from build123d import *

# Parameters (mm, degrees)
CYLINDER713_R     = 1.5
CYLINDER713_DEPTH = 14
CYLINDER710_R     = 1.5
CYLINDER710_DEPTH = 14
CYLINDER711_R     = 1.5
CYLINDER711_DEPTH = 14
CYLINDER712_R     = 1.5
CYLINDER712_DEPTH = 14
BOX045_W          = 15
BOX045_H          = 7.5
BOX045_DEPTH      = 2
BOX044_W          = 15
BOX044_H          = 20
BOX044_DEPTH      = 2
FILLET001008_R    = 3
BOX046_W          = 8
BOX046_H          = 9
BOX046_DEPTH      = 2


with BuildPart() as cylinder783:
    # Cylinder713 → Cylinder713 (new body)
    with BuildSketch(Plane(origin=(-4.5, -50.5, -7), x_dir=(1, 0, 0), z_dir=(0, 0, 1))):
        Circle(CYLINDER713_R)
    extrude(amount=CYLINDER713_DEPTH)


with BuildPart() as fusion001005002004004005002010_body:
    # Cylinder710 → Cylinder710 (new body)
    with BuildSketch(Plane(origin=(4.5, -50.5, -7), x_dir=(1, 0, 0), z_dir=(0, 0, 1))):
        Circle(CYLINDER710_R)
    extrude(amount=CYLINDER710_DEPTH)

    # Fusion001005002004004005002010002003003003017007024017: union Cylinder783
    add(cylinder783.part)


with BuildPart() as fusion001005002004004005002010_body_1:
    # Fusion001005002004004005002010002003003003017007024017 placement: moved
    add(fusion001005002004004005002010_body.part.moved(Location((0, 4, -3))))


with BuildPart() as cylinder781:
    # Cylinder711 → Cylinder711 (new body)
    with BuildSketch(Plane(origin=(-4.5, -50.5, -7), x_dir=(1, 0, 0), z_dir=(0, 0, 1))):
        Circle(CYLINDER711_R)
    extrude(amount=CYLINDER711_DEPTH)


with BuildPart() as fusion001005002004004005002010_body2:
    # Cylinder712 → Cylinder712 (new body)
    with BuildSketch(Plane(origin=(4.5, -50.5, -7), x_dir=(1, 0, 0), z_dir=(0, 0, 1))):
        Circle(CYLINDER712_R)
    extrude(amount=CYLINDER712_DEPTH)

    # Fusion001005002004004005002010002003003003017007024018: union Cylinder781
    add(cylinder781.part)


with BuildPart() as fusion001005002004004005002010_body2_1:
    # Fusion001005002004004005002010002003003003017007024018 placement: moved
    add(fusion001005002004004005002010_body2.part.moved(Location((0, 18, -3))))

    # Fusion001005002004004005002010002003003003017007024019: union Fusion001005002004004005002010 body
    add(fusion001005002004004005002010_body_1.part)


with BuildPart() as cube045:
    # Box045 → Box045 (new body)
    with BuildSketch(Plane(origin=(-7.5, -43.25, -11), x_dir=(1, 0, 0), z_dir=(0, 0, 1))):
        with Locations((7.5, 3.75)):
            Rectangle(BOX045_W, BOX045_H)
    extrude(amount=BOX045_DEPTH)


with BuildPart() as fillet001008:
    # Box044 → Box044 (new body)
    with BuildSketch(Plane(origin=(-7.5, -49.5, -11), x_dir=(1, 0, 0), z_dir=(0, 0, 1))):
        with Locations((7.5, 10)):
            Rectangle(BOX044_W, BOX044_H)
    extrude(amount=BOX044_DEPTH)

    # Cut012030: cut Cube045
    add(cube045.part, mode=Mode.SUBTRACT)

    # Fillet001008
    fillet001008_edges = [fillet001008.edges().sort_by_distance(p)[0] for p in [
        (-7.5, -43.25, -10),
        (-7.5, -49.5, -10),
        (7.5, -43.25, -10),
        (7.5, -49.5, -10),
        (-7.5, -29.5, -10),
        (-7.5, -35.75, -10),
        (7.5, -29.5, -10),
        (7.5, -35.75, -10),
    ]]
    fillet(fillet001008_edges, radius=FILLET001008_R)


with BuildPart() as obj1:
    # Box046 → Box046 (new body)
    with BuildSketch(Plane(origin=(-4, -44, -11), x_dir=(1, 0, 0), z_dir=(0, 0, 1))):
        with Locations((4, 4.5)):
            Rectangle(BOX046_W, BOX046_H)
    extrude(amount=BOX046_DEPTH)

    # Fusion001005002004004005002010002003003003017007024016: union Fillet001008
    add(fillet001008.part)


with BuildPart() as obj1_1:
    # Fusion001005002004004005002010002003003003017007024016 placement: moved
    add(obj1.part.moved(Location((0, 0, 1))))

    # Cut012031: cut Fusion001005002004004005002010 body2
    add(fusion001005002004004005002010_body2_1.part, mode=Mode.SUBTRACT)


with BuildPart() as obj1_2:
    # Cut012031 placement: moved
    add(obj1_1.part.moved(Location((0, 63, 0))))


solid = obj1_2.part
Can you work these out from the model? Positions are in its coordinate system, mm. A direction names the side the tool comes from. Give positions to 0.01 mm unless a question says otherwise; leave off trailing zeros. Order: outer loops, then holes, each group sorted by start corner. A loop starts at its lowest first (then second) coordinate and runs counter-clockwise, first axis right, second up. Notation, with made-up numbers: M -6,22.5 L 4,22.5 A34 cw 4,60.5 Z; hole C 72.5,84 d2. An arc over 180 degrees is marked long. Use one line per item in the form item = value.
Item 1: If I drill on line 1 along X through (y, z) = (30.5, -8.7); line 2 along Y through (x, z) = (-4.5, -9.3), over which ranges is the centre line in solid material (lowest first)? Write a range as [from, to].
Values follow:
line_1 = [-7.5, -6], [-3, 3], [6, 7.5]
line_2 = [13.5, 15], [18, 19.75], [27.25, 29], [32, 33.5]
Item 2: For faces 1 (the flat face through (0, 24, -10)), 2 (the cylindrical face through (6.6, 18.89, -8.99)), 3 (the cylindrical face through (-6.64, 18.85, -8.99)), which set-ups out of +Z, -Z, +X, -X, +Y, -Y let a thin tool reach every point of the face, with its end or its side?
Values follow:
face_1 = -Z, +X, -X, +Y, -Y
face_2 = +Z, -Z, +X
face_3 = +Z, -Z, -X
Item 3: If we section it at A-A, the plane z = -8.8: Write out the boundary of the cut face in (x, y).
Values follow:
outline = M -7.5,16.5 A3 ccw -4.5,13.5 L 4.5,13.5 A3 ccw 7.5,16.5 L 7.5,16.75 A3 ccw 4.5,19.75 L 4,19.75 L 4,27.25 L 4.5,27.25 A3 ccw 7.5,30.25 L 7.5,30.5 A3 ccw 4.5,33.5 L -4.5,33.5 A3 ccw -7.5,30.5 L -7.5,30.25 A3 ccw -4.5,27.25 L -4,27.25 L -4,19.75 L -4.5,19.75 A3 ccw -7.5,16.75 Z; hole C -4.5,16.5 d3; hole C -4.5,30.5 d3; hole C 4.5,16.5 d3; hole C 4.5,30.5 d3
Item 4: Thinking about a two-plate mould opening in X: for faces 4 (the cylindrical face through (-6.64, 32.6, -8.99)), 5 (the cylindrical face through (5.306, 17.765, -9.014)), 6 (the cylindrical face through (-5.61, 17.51, -9.01)), 7 (the flat face through (0, 24, -8)), which applies, pulls with the +X half, pulls with the -X half, needs draft (parallel to the pull), parting line crosses it, or undercut?
Values follow:
face_4 = pulls with the -X half
face_5 = undercut
face_6 = undercut
face_7 = needs draft
Item 5: If we section it at B-B, the plane x = 5.75: Write out the boundary of the cut face in (y, z).
Values follow:
outline = M 13.77,-10 L 15.67,-10 L 15.67,-8 L 13.77,-8 Z; M 17.33,-10 L 19.48,-10 L 19.48,-8 L 17.33,-8 Z; M 27.52,-10 L 29.67,-10 L 29.67,-8 L 27.52,-8 Z; M 31.33,-10 L 33.23,-10 L 33.23,-8 L 31.33,-8 Z
Item 6: If we section it at D-D, the plane y = 26.5: Write out the boundary of the cut face in (x, z).
Values follow:
outline = M -4,-10 L 4,-10 L 4,-8 L -4,-8 Z
Item 7: If we section it at C-C, the plane x = -3.5: Write out the boundary of the cut face in (y, z).
Values follow:
outline = M 13.5,-10 L 15.38,-10 L 15.38,-8 L 13.5,-8 Z; M 17.62,-10 L 29.38,-10 L 29.38,-8 L 17.62,-8 Z; M 31.62,-10 L 33.5,-10 L 33.5,-8 L 31.62,-8 Z
